The model under review builds one solid part; all positions refer to its coordinate system, in mm. A direction names the side the tool comes from. Coordinates: 2 decimals unless noted, no trailing zeros. Order: outer loops, then holes, each group sorted by start corner. A loop starts at its lowest first (then second) coordinate and runs counter-clockwise, first axis right, second up.
```python
from build123d import *

# Parameters (mm, degrees)
F0_R     = 5.05
F1_DEPTH = 6
F0_W     = 21.95
F0_H     = 16
F2_DEPTH = 10.6


with BuildPart() as f1:
    # F0 (on Front) → F1 (new body)
    with BuildSketch(Plane.XZ):
        with Locations((0, 8)):
            Circle(F0_R)
    extrude(amount=F1_DEPTH)

    # F0 (on Front) → F2 (join)
    with BuildSketch(Plane.XZ):
        with Locations((0, 8)):
            Rectangle(F0_W, F0_H)
        with Locations((0, 8)):
            Circle(F0_R, mode=Mode.SUBTRACT)
        with Locations((0, 8)):
            Circle(F0_R)
    extrude(amount=-F2_DEPTH)


solid = f1.part
```
(1) We need section D-D, the plane x = 5.5. Write out the cut boundary in (y, z).
A:
outline: (0, 0) - (10.6, 0) - (10.6, 16) - (0, 16) - close
(2) Draft analysis for pull direction Z (two halves, no side actions). For faces 1 (the face through (0, 10.6, 8)), 2 (the face through (-0.7, -3, 13)), 3 (the face through (0, 5, 16)), state which applies: released by +Z, released by -Z, zero draft, split by the parting line, or undercut.
A:
face 1: zero draft
face 2: split by the parting line
face 3: released by +Z
(3) We need section A-A, the plane x = 0. Write out the cut boundary in (y, z).
A:
outline: (-6, 2.95) - (0, 2.95) - (0, 0) - (10.6, 0) - (10.6, 16) - (0, 16) - (0, 13.05) - (-6, 13.05) - close
(4) We need section C-C, the plane y = -2.5. Write out the cut boundary in (x, z), and give its area (3 significant figures).
A:
outline: circle Ø10.1 at (0, 8)
area: 80.1 mm2
(5) Machinability: for faces 4 (the face through (-5, 0, 10)), 5 (the face through (10.975, 5, 8)), which of the approach directions +Z, -Z, +X, -X, +Y, -Y give a long, thin tool a straight path to every point of the face, cutting with its end or side? Answer none if there is none.
A:
face 4: -Y
face 5: +Z, -Z, +X, +Y, -Y
(6) We need section B-B, the plane z = 14.5. Write out the cut boundary in (x, y) (3 decimals), and give its area (3 significant figures).
A:
outline: (-10.975, 0) - (10.975, 0) - (10.975, 10.6) - (-10.975, 10.6) - close
area: 233 mm2
(7) Wall thickness on probe 1 along Y at (x, z) = (8.5, 9); probe 2 along X at (y, z) = (-0.5, 12); probe 3 along X at (y, z) = (-0.5, 3.75): over which ranges is each line inside the solid? List them lowest first.
A:
probe 1: y = 0 to 10.6
probe 2: x = -3.08 to 3.08
probe 3: x = -2.73 to 2.73
